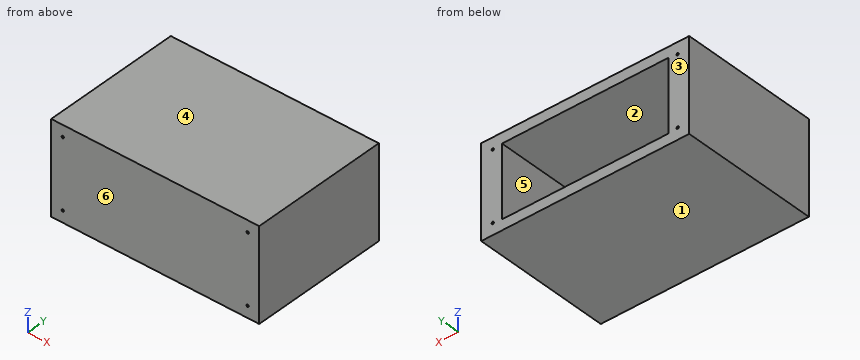
from build123d import *

# Parameters (mm, degrees)
SKETCH4_W           = 228.6
SKETCH4_H           = 101.6
BOSS_EXTRUDE2_DEPTH = 152.4
SKETCH5_W           = 182.88
SKETCH5_H           = 78.74
CUT_EXTRUDE3_DEPTH  = 139.7
SKETCH6_R           = 1.27
CUT_EXTRUDE4_DEPTH  = 153.4


with BuildPart() as part:
    # Sketch4 → Boss-Extrude2 (new body)
    with BuildSketch(Plane(origin=(0, 0, 0), x_dir=(1, 0, 0), z_dir=(0, 1, 0))):
        with Locations((114.3, 50.8)):
            Rectangle(SKETCH4_W, SKETCH4_H)
    extrude(amount=BOSS_EXTRUDE2_DEPTH)

    # Sketch5 → Cut-Extrude3 (cut)
    with BuildSketch(Plane(origin=(0, 152.4, 0), x_dir=(1, 0, 0), z_dir=(0, 1, 0))):
        with Locations((114.3, 50.8)):
            Rectangle(SKETCH5_W, SKETCH5_H)
    extrude(amount=-CUT_EXTRUDE3_DEPTH, mode=Mode.SUBTRACT)

    # Sketch6 → Cut-Extrude4 (cut, through all)
    with BuildSketch(Plane(origin=(0, 152.4, 0), x_dir=(1, 0, 0), z_dir=(0, 1, 0))):
        with Locations((12.7, 88.9)):
            Circle(SKETCH6_R)
        with Locations((215.9, 88.9)):
            Circle(SKETCH6_R)
        with Locations((12.7, 12.7)):
            Circle(SKETCH6_R)
        with Locations((215.9, 12.7)):
            Circle(SKETCH6_R)
    extrude(amount=-CUT_EXTRUDE4_DEPTH, mode=Mode.SUBTRACT)


solid = part.part
Can you work these out from the model? Positions are in its coordinate system, mm. Face numbers are marked on the shaded views. A direction names the side the tool comes from. Give positions to 0.01 mm unless a question says otherwise; leave off trailing zeros. Loops run counter-clockwise (first coordinate to the right, second up) from the corner with the lowest first, then second, coordinate; pieces in that order, holes last. Notation, with made-up numbers: (-8, 21) -> (30, 21) arc R30 cw to (30, 50) -> close; hole circle Ø4 at (72.25, 79.25). An arc over 180 degrees is marked (long way). Write item = value, one per line.
1) Thinking about a two-plate mould opening in Z: for the marked faces 1, 2, 3 and 4, which applies, released by +Z, released by -Z, zero draft, split by the parting line, or undercut?
Check result:
face_1 = released by -Z
face_2 = undercut
face_3 = zero draft
face_4 = released by +Z
2) Suppose I cut it at A-A on y = 33. Write out the boundary of the cut face in (x, z), then the cut area to 3 significant figures.
Check result:
outline = (0, -101.6) -> (228.6, -101.6) -> (228.6, 0) -> (0, 0) -> close; hole circle Ø2.54 at (12.7, -88.9); hole circle Ø2.54 at (12.7, -12.7); hole (22.86, -90.17) -> (205.74, -90.17) -> (205.74, -11.43) -> (22.86, -11.43) -> close; hole circle Ø2.54 at (215.9, -88.9); hole circle Ø2.54 at (215.9, -12.7)
area = 8,810 mm2
3) For the marked faces 5 and 6, which set-ups out of +Z, -Z, +X, -X, +Y, -Y let a thin tool reach every point of the face, with its end or its side?
Check result:
face_5 = +Y
face_6 = +Z, -Z, +X, -X, -Y
4) Suppose I cut it at B-B on x = 149. Write out the boundary of the cut face in (y, z).
Check result:
outline = (0, -101.6) -> (152.4, -101.6) -> (152.4, -90.17) -> (12.7, -90.17) -> (12.7, -11.43) -> (152.4, -11.43) -> (152.4, 0) -> (0, 0) -> close
5) Suppose I cut it at C-C on z = -67.5. Write out the boundary of the cut face in (x, y), then the cut area to 3 significant figures.
Check result:
outline = (0, 0) -> (228.6, 0) -> (228.6, 152.4) -> (205.74, 152.4) -> (205.74, 12.7) -> (22.86, 12.7) -> (22.86, 152.4) -> (0, 152.4) -> close
area = 9,290 mm2
6) Will this pin go through, and if not, where does the flat tip stop? pin 1 (8 mm diameter, centred on x = 149, z = -51.5, fed in from +Y).
Check result:
pin_1 = 12.7
7) I need wall thicknesses on L1, parallel to Z at x = 215.9, y = 95; L2, parallel to X at y = 55, z = -12.7; L3, parallel to Z at x = 84, y = 95.5. Which ranges of each line are inside material? Lowest first, please. Write a range as from..to.
Check result:
L1 = -101.6..-90.17, -87.63..-13.97, -11.43..0
L2 = 0..11.43, 13.97..22.86, 205.74..214.63, 217.17..228.6
L3 = -101.6..-90.17, -11.43..0
